Study the drawing (mm; zero at the part's minimum x, y, z) and answer. A direction names the side the tool comes from. Round coordinates to 2 decimals unless told otherwise and drop trailing zeros. Order: outer loops, then holes, each group sorted by start corner. A loop starts at its lowest first (then second) coordinate and runs counter-clockwise, first axis right, second up. Notation, with made-up numbers: (-6, -33) - (13, -33) arc R20 cw to (13, -8) - close; hole circle Ø1 at (6.25, -20). An arc over 180 degrees is marked (long way). Put each result on its own line as item: value. Start each with the question number.
Q1. Each of these flat-tipped pins is pushed along its axis until it touches: pin 1 Ø3.5 at (x, y) = (36.65, 28.5) entering from +Z; pin 2 Ø17 at (x, y) = (16, 36) entering from -Z; pin 3 Ø6.5 at (x, y) = (26.5, 17) entering from -Z. Where does it stop, or does it pass through?
Q2. Section D-D on y = 13 is taken. Give the vertices of the cut face in (x, z).
Q3. Find the intervals of material crossed by line 1 along X through (y, z) = (11, 30.5); line 2 along X through (y, z) = (28, 75); line 3 along X through (y, z) = (28, 72), in increasing order. Write a range as from..to.
Q4. Which of the six approach directions +Z, -Z, +X, -X, +Y, -Y give full straight-line access (tool end or side, diameter ignored) to the marked faces 1, 2 and 3?
Q5. Section A-A on z = 63.1 is taken. Give the vertices of the cut face in (x, y).
Q6. Section B-B on x = 36.65 is taken. Give the vertices of the cut face in (y, z).
Q7. Section C-C on y = 33 is taken. Give the vertices of the cut face in (x, z), then the cut area to 3 significant figures.
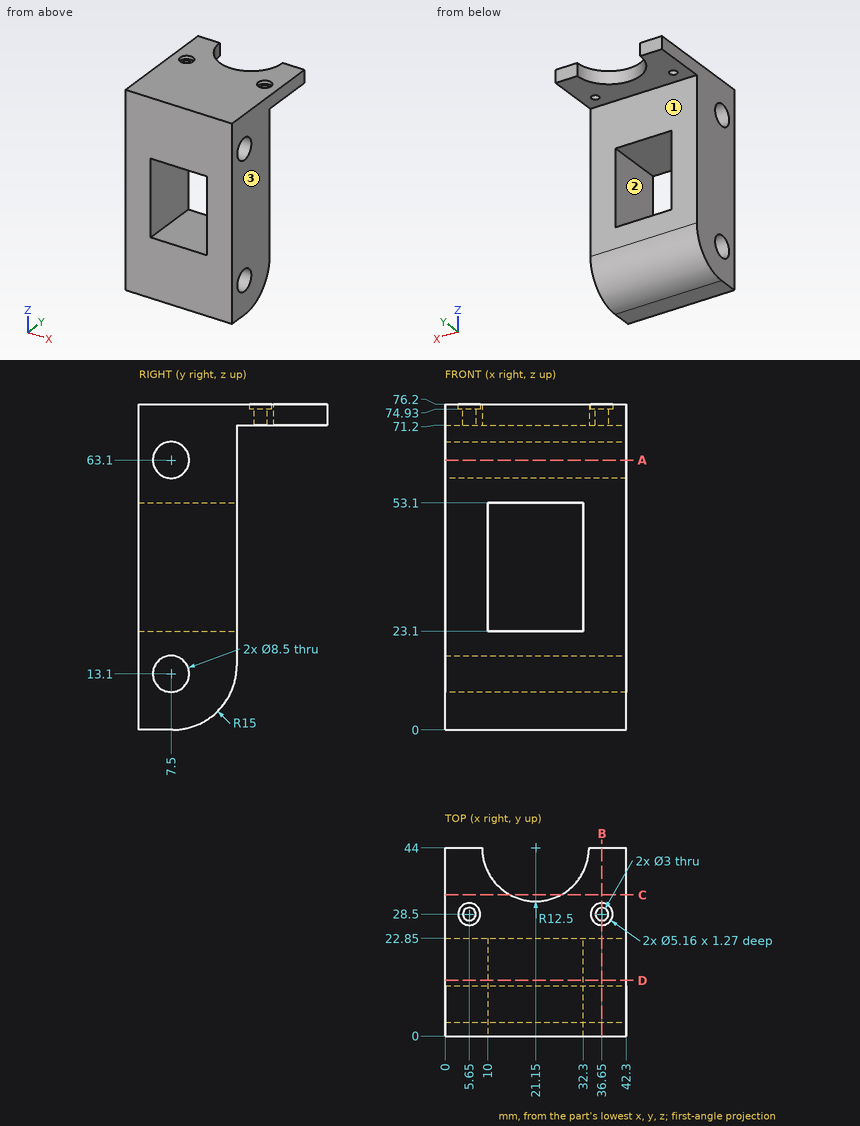
Findings:
1. pin 1: z = 74.93
1. pin 2: z = 71.2
1. pin 3: z = 1.21
2. outline: (0, 0.91) - (42.3, 0.91) - (42.3, 76.2) - (0, 76.2) - close; hole (10, 23.1) - (32.3, 23.1) - (32.3, 53.1) - (10, 53.1) - close
3. line 1: 0..10, 32.3..42.3
3. line 2: 0..3.12, 8.18..34.12, 39.18..42.3
3. line 3: 0..4.24, 7.06..35.24, 38.06..42.3
4. face 1: -Z, +X, -X, +Y
4. face 2: +Y, -Y
4. face 3: +Z, -Z, +X, +Y, -Y
5. outline: (0, 0) - (42.3, 0) - (42.3, 3.25) - (0, 3.25) - close; (0, 11.75) - (42.3, 11.75) - (42.3, 22.85) - (0, 22.85) - close
6. outline: (0, 0) - (7.85, 0) arc R15 ccw to (22.85, 15) - (22.85, 71.2) - (27, 71.2) - (27, 74.93) - (25.92, 74.93) - (25.92, 76.2) - (0, 76.2) - close; (30, 71.2) - (44, 71.2) - (44, 76.2) - (31.08, 76.2) - (31.08, 74.93) - (30, 74.93) - close; hole circle Ø8.5 at (7.5, 13.1); hole circle Ø8.5 at (7.5, 63.1)
7. outline: (0, 71.2) - (15.21, 71.2) - (15.21, 76.2) - (0, 76.2) - close; (27.09, 71.2) - (42.3, 71.2) - (42.3, 76.2) - (27.09, 76.2) - close
7. area: 152 mm2
